Geometry check sheet. Reference: drawing and pictorial views, mm from the part's lowest x, y, z. Round coordinates to 2 decimals unless told otherwise and drop trailing zeros. Write each loop counter-clockwise with the first axis right and the second up, starting at its lowest first coordinate (ties: lowest second). Pieces come first, ordered by that corner, then holes. Notation, with made-up numbers: (-16, 30.5) - (21, 30.5) arc R19 cw to (21, 40.5) - close; hole circle Ø4 at (-39.5, 35). An arc over 180 degrees is marked (long way). Use one line per item in the form item = value. Start each with the question number.
1) Section check C-C (x = 10). Record the boundary of the cut face in (y, z).
2) Section check A-A (y = 1.75). Record the boundary of the cut face in (x, z), then the cut area to 3 significant figures.
3) Section check B-B (z = 3.75). Record the boundary of the cut face in (x, y) (1 decimal).
4) Scan lines: probe 1 along Z at (x, y) = (1, 2.2); probe 2 along X at (y, z) = (0.4, 9.75) (1 decimal); probe 3 along X at (y, z) = (2.7, 6.5) (1 decimal). Record each from-to range of solid material in increasing order.
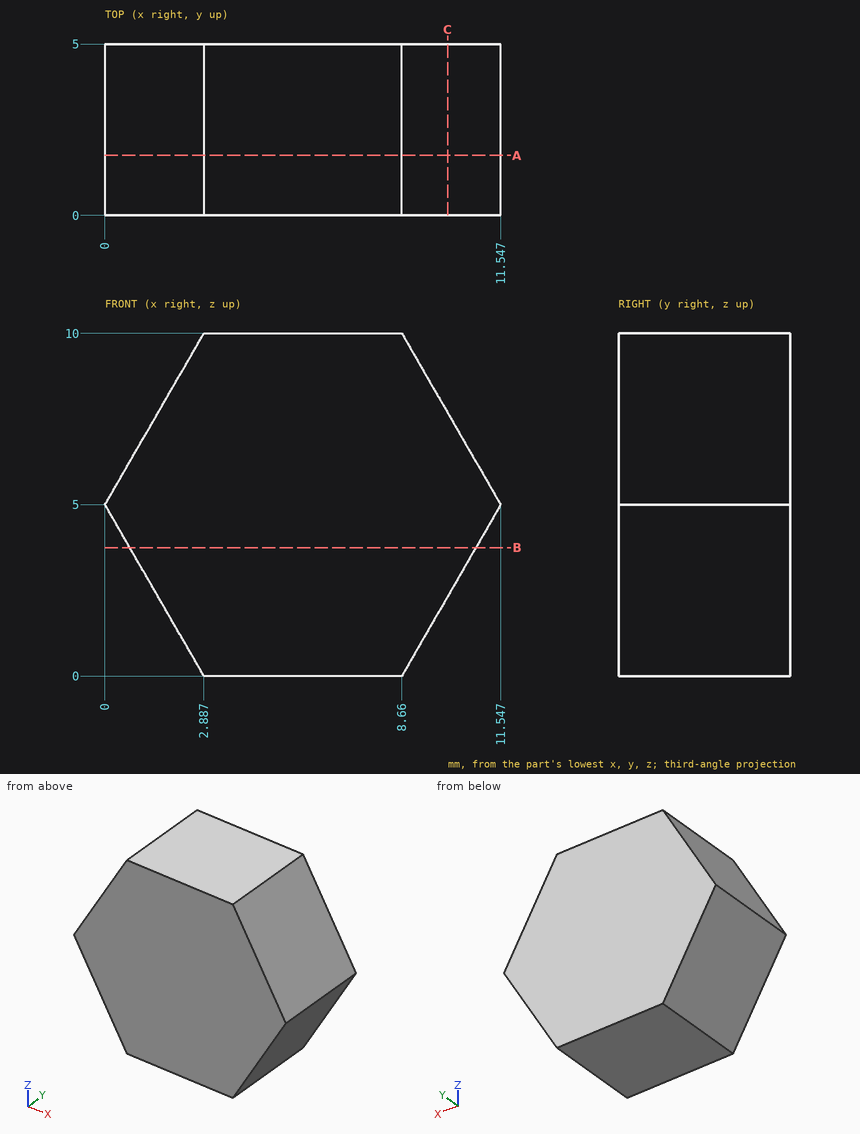
Results are:
q1.outline = (0, 2.32) - (5, 2.32) - (5, 7.68) - (0, 7.68) - close
q2.outline = (0, 5) - (2.89, 0) - (8.66, 0) - (11.55, 5) - (8.66, 10) - (2.89, 10) - close
q2.area = 86.6 mm²
q3.outline = (0.7, 0) - (10.8, 0) - (10.8, 5) - (0.7, 5) - close
q4.probe_1 = 3.27 to 6.73
q4.probe_2 = 2.7 to 8.8
q4.probe_3 = 0.9 to 10.7
